The model under review builds one solid part; all positions refer to its coordinate system, in mm. Face numbers are marked on the shaded views. A direction names the side the tool comes from. Coordinates: 2 decimals unless noted, no trailing zeros. Write each loop counter-clockwise with the first axis right and the second up, starting at its lowest first coordinate (ties: lowest second). Pieces come first, ordered by that corner, then holes. Notation, with made-up numbers: M 42,62 L 95,62 A20 cw 95,93 Z; hole C 5,21 d8. An arc over 180 degrees is marked long. Answer as a JSON object with one key per item and string values.
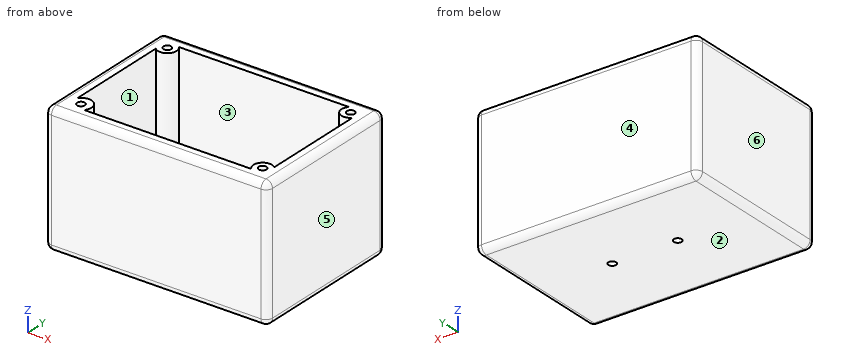
```python
from build123d import *

# Parameters (mm, degrees)
F0_W     = 170
F0_H     = 100
F1_DEPTH = 60
F2_T     = -10
F3_R     = 5
F4_R     = 3
F5_DEPTH = 90
F7_D     = 6


with BuildPart() as f1:
    # F0 (on Front) → F1 (new body, symmetric)
    with BuildSketch(Plane.XZ):
        Rectangle(F0_W, F0_H)
    extrude(amount=F1_DEPTH, both=True)

    # F2
    f2_openings = [f1.faces().sort_by_distance(p)[0] for p in [
        (0, 0, 50),
    ]]
    offset(amount=F2_T, openings=f2_openings)

    # F3
    f3_edges = [f1.edges().sort_by_distance(p)[0] for p in [
        (-85, 0, 50),
        (0, -60, 50),
        (85, 0, 50),
        (0, 60, 50),
        (85, 60, 0),
        (85, -60, 0),
        (85, 0, -50),
        (-85, -60, 0),
        (0, -60, -50),
        (-85, 60, 0),
        (-85, 0, -50),
        (0, 60, -50),
    ]]
    fillet(f3_edges, radius=F3_R)

    # F4 (on face) → F5 (join, through all)
    with BuildSketch(Plane.XY.offset(50)):
        with BuildLine():
            Line((-65, 50), (-75, 50))
            Line((-75, 50), (-75, 40))
            ThreePointArc((-75, 40), (-65, 40), (-65, 50))
        make_face()
        with Locations((-70, 45)):
            Circle(F4_R, mode=Mode.SUBTRACT)
        with BuildLine():
            Line((75, 40), (75, 50))
            Line((75, 50), (65, 50))
            ThreePointArc((65, 50), (65, 40), (75, 40))
        make_face()
        with Locations((70, 45)):
            Circle(F4_R, mode=Mode.SUBTRACT)
        with BuildLine():
            Line((65, -50), (75, -50))
            Line((75, -50), (75, -40))
            ThreePointArc((75, -40), (65, -40), (65, -50))
        make_face()
        with Locations((70, -45)):
            Circle(F4_R, mode=Mode.SUBTRACT)
        with BuildLine():
            Line((-75, -40), (-75, -50))
            Line((-75, -50), (-62.405661, -50))
            ThreePointArc((-62.405661, -50), (-63.70283, -38.70283), (-75, -40))
        make_face()
        with Locations((-68.70283, -45)):
            Circle(F4_R, mode=Mode.SUBTRACT)
    extrude(amount=-F5_DEPTH)

    # F7 (through all)
    with Locations(Plane(origin=(0, 0, -50), x_dir=(1, 0, 0), z_dir=(0, 0, -1))):
        with Locations((-25, 0), (25, 0)):
            Hole(F7_D / 2)


solid = f1.part
```
(1) For pin 1 Ø3 at (x, y) = (-70.5, 45) entering from +Z; pin 2 Ø6.5 at (x, y) = (-68, -45) entering from +Z, all flat-tipped, find the tip position at first contact; note any pin that passes through.
Results list:
{"pin 1": "z = -40", "pin 2": "z = 50"}
(2) Add section C-C on y = -10. Give the boundary of the cut face in (x, z), and give its area (3 significant figures).
Results list:
{"outline": "M -85,-45 A5 ccw -80,-50 L 80,-50 A5 ccw 85,-45 L 85,45 A5 ccw 80,50 L 75,50 L 75,-40 L -75,-40 L -75,50 L -80,50 A5 ccw -85,45 Z", "area": "3,480 mm²"}
(3) Draft analysis for pull direction X (two halves, no side actions). For the marked faces 3, 4, 5 and 6, state which applies: released by +X, released by -X, zero draft, split by the parting line, or undercut.
Results list:
{"face 3": "undercut", "face 4": "zero draft", "face 5": "released by +X", "face 6": "released by -X"}
(4) Wall thickness on line 1 along Y through (x, z) = (70, -12); line 2 along Y through (x, z) = (-47, 43); line 3 along X through (y, z) = (21.5, -10.5): over which ranges is each line inside the solid? List them lowest first. Write a range as from..to.
Results list:
{"line 1": "-60..-48, -42..-37.93, 37.93..42, 48..60", "line 2": "-60..-50, 50..60", "line 3": "-85..-75, 75..85"}
(5) Add section B-B on z = 30.5. Give the boundary of the cut face in (x, y), and give its area (3 significant figures).
Results list:
{"outline": "M -85,-55 A5 ccw -80,-60 L 80,-60 A5 ccw 85,-55 L 85,55 A5 ccw 80,60 L -80,60 A5 ccw -85,55 Z; hole M -75,-40 A8.04 cw -62.41,-50 L 65,-50 A7.07 cw 75,-40 L 75,40 A7.07 cw 65,50 L -65,50 A7.07 cw -75,40 Z; hole C -70,45 d6; hole C -68.7,-45 d6; hole C 70,-45 d6; hole C 70,45 d6", "area": "5,820 mm²"}
(6) For the marked faces 1 and 2, list the 3-axis set-ups (+Z, -Z, +X, -X, +Y, -Y) from which the entire face can be reached by the end or side of a thin tool; tool diameter is ignored.
Results list:
{"face 1": "+Z", "face 2": "-Z, +X, -X, +Y, -Y"}
(7) Add section D-D on x = -51. Give the boundary of the cut face in (y, z), and give its area (3 significant figures).
Results list:
{"outline": "M -60,-45 A5 ccw -55,-50 L 55,-50 A5 ccw 60,-45 L 60,45 A5 ccw 55,50 L 50,50 L 50,-40 L -50,-40 L -50,50 L -55,50 A5 ccw -60,45 Z", "area": "2,980 mm²"}
(8) Add section A-A on x = -25. Give the boundary of the cut face in (y, z), and give its area (3 significant figures).
Results list:
{"outline": "M -60,-45 A5 ccw -55,-50 L -3,-50 L -3,-40 L -50,-40 L -50,50 L -55,50 A5 ccw -60,45 Z; M 3,-50 L 55,-50 A5 ccw 60,-45 L 60,45 A5 ccw 55,50 L 50,50 L 50,-40 L 3,-40 Z", "area": "2,920 mm²"}
